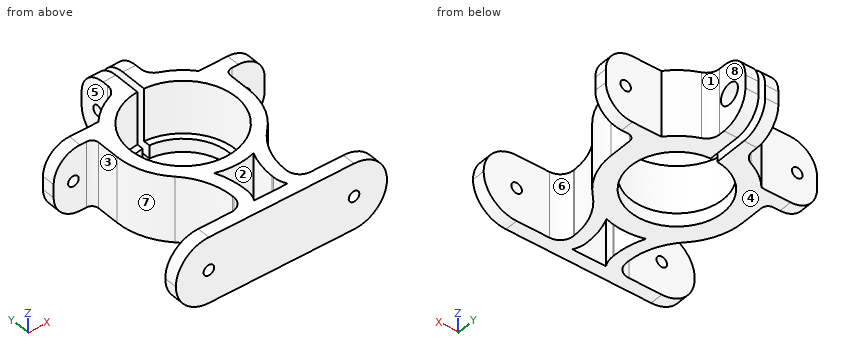
from build123d import *

# Parameters (mm, degrees)
BOSS_EXTRUDE1_DEPTH = 10
SKETCH3_R           = 0.8
CUT_EXTRUDE1_DEPTH  = 2
SKETCH4_R           = 0.8
CUT_EXTRUDE2_DEPTH  = 2
SKETCH5_R           = 0.8
CUT_EXTRUDE3_DEPTH  = 2
SKETCH6_R           = 0.8
CUT_EXTRUDE4_DEPTH  = 3
SKETCH7_R           = 1.6
CUT_EXTRUDE5_DEPTH  = 3
CUT_EXTRUDE6_DEPTH  = 10
BOSS_EXTRUDE2_DEPTH = 2


with BuildPart() as part:
    # Sketch1 → Boss-Extrude1 (new body)
    with BuildSketch(Plane.XY):
        with BuildLine():
            Line((16.803004448, 0), (48.803096805, 0))
            Line((48.803096805, 0), (48.803096805, 2))
            Line((48.803096805, 2), (38.803096805, 2))
            ThreePointArc((38.803096805, 2), (37.388883243, 2.585786438), (36.803096805, 4))
            Line((36.803096805, 4), (36.803096805, 4.217123744))
            ThreePointArc((36.803096805, 4.217123744), (37.58355047, 8.090102619), (39.803089878, 11.358545383))
            ThreePointArc((39.803089878, 11.358545383), (42.022639537, 14.62700324), (42.803096805, 18.5))
            Line((42.803096805, 18.5), (42.803096805, 22))
            ThreePointArc((42.803096805, 22), (43.095990024, 22.707106781), (43.803096805, 23))
            Line((43.803096805, 23), (48.803096805, 23))
            Line((48.803096805, 23), (48.803096805, 25))
            Line((48.803096805, 25), (44.105786895, 25))
            Line((44.105786895, 25), (40.40245347, 25))
            ThreePointArc((40.40245347, 25), (38.644426823, 26.616603213), (36.553207437, 27.770234489))
            ThreePointArc((36.553207437, 27.770234489), (35.644914528, 28.506251313), (35.303235335, 29.624272825))
            Line((35.303235335, 29.624272825), (35.303235335, 34.487492178))
            Line((35.303235335, 34.487492178), (33.303050626, 34.487492178))
            Line((33.303050626, 34.487492178), (33.303050626, 26.484348185))
            ThreePointArc((33.303050626, 26.484348185), (32.803050626, 10.500011503), (32.303050626, 26.484348185))
            Line((32.303050626, 26.484348185), (32.303050626, 34.487492178))
            Line((32.303050626, 34.487492178), (30.303050626, 34.487492178))
            Line((30.303050626, 34.487492178), (30.303050626, 29.624347545))
            ThreePointArc((30.303050626, 29.624347545), (29.961362151, 28.506312265), (29.05304774, 27.770296755))
            ThreePointArc((29.05304774, 27.770296755), (26.961741815, 26.616651708), (25.203647783, 25))
            Line((25.203647783, 25), (21.500314358, 25))
            Line((21.500314358, 25), (16.803004448, 25))
            Line((16.803004448, 25), (16.803004448, 23))
            Line((16.803004448, 23), (21.803004448, 23))
            ThreePointArc((21.803004448, 23), (22.510111229, 22.707106781), (22.803004448, 22))
            Line((22.803004448, 22), (22.803004448, 18.5))
            ThreePointArc((22.803004448, 18.5), (23.583461716, 14.62700324), (25.803011375, 11.358545383))
            ThreePointArc((25.803011375, 11.358545383), (28.022550783, 8.090102619), (28.803004448, 4.217123744))
            Line((28.803004448, 4.217123744), (28.803004448, 4))
            ThreePointArc((28.803004448, 4), (28.21721801, 2.585786438), (26.803004448, 2))
            Line((26.803004448, 2), (16.803004448, 2))
            Line((16.803004448, 2), (16.803004448, 0))
        make_face()
        with BuildLine():
            Line((34.803096805, 4), (34.803096805, 4.217123744))
            ThreePointArc((34.803096805, 4.217123744), (35.049071096, 6.634328662), (35.776910074, 8.952438536))
            ThreePointArc((35.776910074, 8.952438536), (32.803050626, 8.500011503), (29.829191179, 8.952438536))
            ThreePointArc((29.829191179, 8.952438536), (30.557030157, 6.634328662), (30.803004448, 4.217123744))
            Line((30.803004448, 4.217123744), (30.803004448, 4))
            ThreePointArc((30.803004448, 4), (30.666707753, 2.96472382), (30.267106063, 2))
            Line((30.267106063, 2), (35.33899519, 2))
            ThreePointArc((35.33899519, 2), (34.9393935, 2.96472382), (34.803096805, 4))
        make_face(mode=Mode.SUBTRACT)
    extrude(amount=BOSS_EXTRUDE1_DEPTH)

    # Sketch3 → Cut-Extrude1 (cut)
    with BuildSketch(Plane(origin=(0, 2, 0), x_dir=(1, 0, 0), z_dir=(0, 1, 0))):
        with BuildLine():
            ThreePointArc((48.803096805, -5), (47.338630711, -8.535533906), (43.803096805, -10))
            Line((43.803096805, -10), (48.803096805, -10))
            Line((48.803096805, -10), (48.803096805, -5))
        make_face()
        with BuildLine():
            ThreePointArc((43.803096805, 0), (47.338630711, -1.464466094), (48.803096805, -5))
            Line((48.803096805, -5), (48.803096805, 0))
            Line((48.803096805, 0), (43.803096805, 0))
        make_face()
        with Locations(Location((43.803096805, -5, 0), (0, 0, 180))):
            Circle(SKETCH3_R)
    extrude(amount=-CUT_EXTRUDE1_DEPTH, mode=Mode.SUBTRACT)

    # Sketch4 → Cut-Extrude2 (cut)
    with BuildSketch(Plane(origin=(0, 2, 0), x_dir=(1, 0, 0), z_dir=(0, 1, 0))):
        with BuildLine():
            Line((16.803004448, -10), (21.803004448, -10))
            ThreePointArc((21.803004448, -10), (18.267470542, -8.535533906), (16.803004448, -5))
            Line((16.803004448, -5), (16.803004448, -10))
        make_face()
        with BuildLine():
            Line((16.803004448, 0), (16.803004448, -5))
            ThreePointArc((16.803004448, -5), (18.267470542, -1.464466094), (21.803004448, 0))
            Line((21.803004448, 0), (16.803004448, 0))
        make_face()
        with Locations(Location((21.803004448, -5, 0), (0, 0, 270))):
            Circle(SKETCH4_R)
    extrude(amount=-CUT_EXTRUDE2_DEPTH, mode=Mode.SUBTRACT)

    # Sketch5 → Cut-Extrude3 (cut)
    with BuildSketch(Plane(origin=(0, 25, 0), x_dir=(1, 0, 0), z_dir=(0, 1, 0))):
        with Locations(Location((19.803004448, -5, 0), (0, 0, 270))):
            Circle(SKETCH5_R)
        with Locations(Location((45.803096805, -5, 0), (0, 0, 270))):
            Circle(SKETCH5_R)
        with BuildLine():
            Line((20.803004448, -10), (16.803004448, -10))
            Line((16.803004448, -10), (16.803004448, -6))
            ThreePointArc((16.803004448, -6), (17.974577323, -8.828427125), (20.803004448, -10))
        make_face()
        with BuildLine():
            Line((16.803004448, -4), (16.803004448, 0))
            Line((16.803004448, 0), (20.803004448, 0))
            ThreePointArc((20.803004448, 0), (17.974577323, -1.171572875), (16.803004448, -4))
        make_face()
        with BuildLine():
            Line((44.803096805, 0), (48.803096805, 0))
            Line((48.803096805, 0), (48.803096805, -4))
            ThreePointArc((48.803096805, -4), (47.63152393, -1.171572875), (44.803096805, 0))
        make_face()
        with BuildLine():
            Line((48.803096805, -6), (48.803096805, -10))
            Line((48.803096805, -10), (44.803096805, -10))
            ThreePointArc((44.803096805, -10), (47.63152393, -8.828427125), (48.803096805, -6))
        make_face()
    extrude(amount=-CUT_EXTRUDE3_DEPTH, mode=Mode.SUBTRACT)

    # Sketch6 → Cut-Extrude4 (cut)
    with BuildSketch(Plane.ZY.offset(-30.303050626)):
        with Locations((5, 31.487492178)):
            Circle(SKETCH6_R)
    extrude(amount=-CUT_EXTRUDE4_DEPTH, mode=Mode.SUBTRACT)

    # Sketch7 → Cut-Extrude5 (cut)
    with BuildSketch(Plane(origin=(35.303235335, 0, 0), x_dir=(0, 0, -1), z_dir=(1, 0, 0))):
        with Locations((-5, 31.487492178)):
            Circle(SKETCH7_R)
    extrude(amount=-CUT_EXTRUDE5_DEPTH, mode=Mode.SUBTRACT)

    # Sketch8 → Cut-Extrude6 (cut)
    with BuildSketch(Plane.ZY.offset(-30.303050626)):
        with BuildLine():
            Line((0, 30.487492178), (0, 34.487492178))
            Line((0, 34.487492178), (4, 34.487492178))
            ThreePointArc((4, 34.487492178), (1.171572875, 33.315919302), (0, 30.487492178))
        make_face()
        with BuildLine():
            Line((6, 34.487492178), (10, 34.487492178))
            Line((10, 34.487492178), (10, 30.487492178))
            ThreePointArc((10, 30.487492178), (8.828427125, 33.315919302), (6, 34.487492178))
        make_face()
    extrude(amount=-CUT_EXTRUDE6_DEPTH, mode=Mode.SUBTRACT)

    # Sketch9 → Boss-Extrude2 (add)
    with BuildSketch(Plane(origin=(0, 0, 0), x_dir=(-1, 0, 0), z_dir=(0, 0, -1))):
        with BuildLine():
            Line((-33.303050626, 26.484348185), (-33.303050626, 25.482120022))
            ThreePointArc((-33.303050626, 25.482120022), (-32.803050626, 11.5), (-32.303050626, 25.482120022))
            Line((-32.303050626, 25.482120022), (-32.303050626, 26.484348185))
            ThreePointArc((-32.303050626, 26.484348185), (-32.803050626, 10.500011503), (-33.303050626, 26.484348185))
        make_face()
    extrude(amount=-BOSS_EXTRUDE2_DEPTH)


solid = part.part
Part model, mm, in its own coordinate system. Face numbers are marked on the shaded views. A direction names the side the tool comes from. Give positions to 0.01 mm unless a question says otherwise; leave off trailing zeros. Loops run counter-clockwise (first coordinate to the right, second up) from the corner with the lowest first, then second, coordinate; pieces in that order, holes last. Notation, with made-up numbers: (-16.5, -4.5) -> (-2.5, -4.5) arc R15 ccw to (-2.5, 16.5) -> close; hole circle Ø5 at (70, -34). An arc over 180 degrees is marked (long way). Write each question's results on one line, items separated by ' | '. Start each with the question number.
Q1. Band-saw the part on A-A on x = 31.5. List the corners of the cut face in (y, z).
Q2. Which spindle directions (+Z, -Z, +X, -X, +Y, -Y) get a long thin tool onto all of the face, cutting with end or side? Do the marked faces 4, 5, 6, 7 and 8. Say none if no direction does.
Q3. Pin check, flat tips, straight feed: P1, Ø4, axis at y = 20.5, z = 5, coming from the -X side; P2, Ø1.5, axis at y = 15.5, z = 5.5, coming from the +X side; P3, Ø5, axis at y = 28.5, z = 9, coming from the -X side. Stop position of each tip, or through.
Q4. Band-saw the part on D-D on y = 20. List the corners of the cut face in (x, z).
Q5. Wall check: L1, parallel to Y at x = 18, z = 3.5; L2, parallel to X at y = 18.5, z = 0.55; L3, parallel to X at y = 18.5, z = 4.25. Give the ranges that are in metal, low to high.
Q6. Pull direction X, two halves, no side cores. Call the marked faces 1, 2 and 3: +X half, -X half, draft (parallel to the pull), parting line (faces both ways), or undercut.
Q7. Band-saw the part on B-B on y = 8. List the corners of the cut face in (x, z), plus the area to 3 significant figures.
Q8. Band-saw the part on C-C on x = 24. List the corners of the cut face in (y, z), plus the area to 3 significant figures.
Results are:
1) outline: (0, 0) -> (2, 0) -> (2, 10) -> (0, 10) -> close; (8.59, 0) -> (11.62, 0) -> (11.62, 2) -> (10.61, 2) -> (10.61, 10) -> (8.59, 10) -> close; (25.38, 0) -> (30.49, 0) arc R4 ccw to (34.49, 4) -> (34.49, 6) arc R4 ccw to (30.49, 10) -> (26.39, 10) -> (26.39, 2) -> (25.38, 2) -> close; hole circle Ø1.6 at (31.49, 5)
2) face 4: -Z, +X, -X, +Y, -Y | face 5: +Z, -Z, -X, +Y | face 6: +Z, -Z, +X | face 7: +Z, -Z, -X | face 8: +Z, -Z, +X, +Y
3) P1: stops at x = 22.67 | P2: stops at x = 42.55 | P3: stops at x = 26.19
4) outline: (22.8, 0) -> (25.97, 0) -> (25.97, 2) -> (24.94, 2) -> (24.94, 10) -> (22.8, 10) -> close; (39.64, 0) -> (42.8, 0) -> (42.8, 10) -> (40.66, 10) -> (40.66, 2) -> (39.64, 2) -> close
5) L1: y = 0 to 2, 23 to 25 | L2: x = 22.8 to 25.8, 39.8 to 42.8 | L3: x = 22.8 to 24.8, 40.8 to 42.8
6) face 1: +X half | face 2: undercut | face 3: -X half
7) outline: (28.06, 0) -> (30.19, 0) -> (30.19, 10) -> (28.06, 10) -> close; (35.41, 0) -> (37.55, 0) -> (37.55, 10) -> (35.41, 10) -> close | area: 42.6 mm²
8) outline: (0, 0) -> (2, 0) -> (2, 10) -> (0, 10) -> close; (13.76, 0) -> (25, 0) -> (25, 10) -> (13.76, 10) -> close | area: 132 mm²
